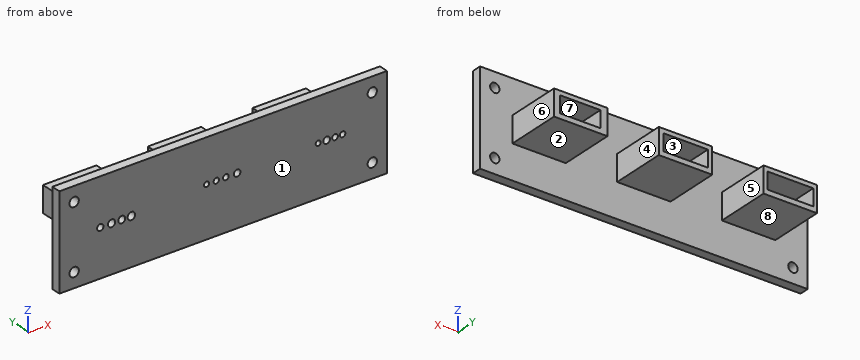
```python
from build123d import *

# Parameters (mm, degrees)
SKETCH1_W           = 88.9
SKETCH1_H           = 25.4
BOSS_EXTRUDE1_DEPTH = 2.54
SKETCH2_R           = 1.27
CUT_EXTRUDE1_DEPTH  = 2.54
SKETCH16_W          = 14.499999956
SKETCH16_H          = 6.99999997
BOSS_EXTRUDE3_DEPTH = 14.999999972
SKETCH17_W          = 12.390836481
SKETCH17_H          = 4.505758721
SKETCH17_W_2        = 12.015356588
SKETCH17_W_3        = 10.95149689
CUT_EXTRUDE4_DEPTH  = 12.459999972
SKETCH18_R          = 0.865438392
SKETCH18_R_2        = 0.972006337
SKETCH18_R_3        = 0.938699733
SKETCH18_R_4        = 1.023043952
SKETCH18_R_5        = 0.699865796
SKETCH18_R_6        = 0.72485584
SKETCH18_R_7        = 0.753208606
SKETCH18_R_8        = 0.89391984
SKETCH18_R_9        = 0.684371717
SKETCH18_R_10       = 0.906595882
SKETCH18_R_11       = 0.774291856
SKETCH18_R_12       = 0.739788643
CUT_EXTRUDE5_DEPTH  = 12.459999972


with BuildPart() as part:
    # Sketch1 → Boss-Extrude1 (new body)
    with BuildSketch(Plane(origin=(0, 0, 0), x_dir=(1, 0, 0), z_dir=(0, 1, 0))):
        Rectangle(SKETCH1_W, SKETCH1_H)
    extrude(amount=BOSS_EXTRUDE1_DEPTH)

    # Sketch2 → Cut-Extrude1 (cut)
    with BuildSketch(Plane(origin=(0, 2.54, 0), x_dir=(1, 0, 0), z_dir=(0, 1, 0))):
        with Locations((-40.45, 8.7)):
            Circle(SKETCH2_R)
        with Locations((-40.45, -8.7)):
            Circle(SKETCH2_R)
        with Locations((40.45, -8.7)):
            Circle(SKETCH2_R)
        with Locations((40.45, 8.7)):
            Circle(SKETCH2_R)
    extrude(amount=-CUT_EXTRUDE1_DEPTH, mode=Mode.SUBTRACT)

    # Sketch16 → Boss-Extrude3 (add)
    with BuildSketch(Plane(origin=(0, 2.54, 0), x_dir=(1, 0, 0), z_dir=(0, 1, 0))):
        Rectangle(SKETCH16_W, SKETCH16_H)
        with Locations((28.430000036, 1.27e-07)):
            Rectangle(SKETCH16_W, SKETCH16_H)
        with Locations((-28.430000036, 1.27e-07)):
            Rectangle(SKETCH16_W, SKETCH16_H)
    extrude(amount=BOSS_EXTRUDE3_DEPTH)

    # Sketch17 → Cut-Extrude4 (cut)
    with BuildSketch(Plane(origin=(0, 17.539999972, 0), x_dir=(1, 0, 0), z_dir=(0, 1, 0))):
        with Locations((-28.473891916, -0.093869973)):
            Rectangle(SKETCH17_W, SKETCH17_H)
        with Locations((-0.062579982, -0.093869973)):
            Rectangle(SKETCH17_W_2, SKETCH17_H)
        with Locations((28.567761889, -0.093869973)):
            Rectangle(SKETCH17_W_3, SKETCH17_H)
    extrude(amount=-CUT_EXTRUDE4_DEPTH, mode=Mode.SUBTRACT)

    # Sketch18 → Cut-Extrude5 (cut)
    with BuildSketch(Plane(origin=(0, 5.08, 0), x_dir=(1, 0, 0), z_dir=(0, 1, 0))):
        with Locations((-33.35513053, 0)):
            Circle(SKETCH18_R)
        with Locations((-30.2887114, 0)):
            Circle(SKETCH18_R_2)
        with Locations((-27.535192182, 0)):
            Circle(SKETCH18_R_3)
        with Locations((-24.906832928, 0)):
            Circle(SKETCH18_R_4)
        with Locations((-4.506191176, -1.023043952)):
            Circle(SKETCH18_R_5)
        with Locations((-1.873685579, -1.023043952)):
            Circle(SKETCH18_R_6)
        with Locations((0.727684736, -1.023043952)):
            Circle(SKETCH18_R_7)
        with Locations((3.790367697, -1.023043952)):
            Circle(SKETCH18_R_8)
        with Locations((25.783303286, -1.023043952)):
            Circle(SKETCH18_R_9)
        with Locations((28.074005802, -1.023043952)):
            Circle(SKETCH18_R_10)
        with Locations((30.354212641, -1.023043952)):
            Circle(SKETCH18_R_11)
        with Locations((32.413417846, -1.023043952)):
            Circle(SKETCH18_R_12)
    extrude(amount=-CUT_EXTRUDE5_DEPTH, mode=Mode.SUBTRACT)


solid = part.part
```
The model under review builds one solid part; all positions refer to its coordinate system, in mm. Face numbers are marked on the shaded views. A direction names the side the tool comes from. Coordinates: 2 decimals unless noted, no trailing zeros. Order: outer loops, then holes, each group sorted by start corner. A loop starts at its lowest first (then second) coordinate and runs counter-clockwise, first axis right, second up. Notation, with made-up numbers: (6.5, -33.75) -> (17.5, -33.75) arc R18 ccw to (17.5, -8.75) -> close; hole circle Ø11 at (-37, 55). An arc over 180 degrees is marked (long way). Answer in a Markdown table with one row per item. Add a question column.
Item 1: We need section D-D on x = 11. Write out the cut boundary in (y, z), plus the area to 3 significant figures.
Item 2: Machinability: for the marked faces 1, 2, 3 and 4, which of the approach directions +Z, -Z, +X, -X, +Y, -Y give a long, thin tool a straight path to every point of the face, cutting with its end or side? Answer none if there is none.
Item 3: We need section C-C on z = -8.7. Write out the cut boundary in (x, y), plus the area to 3 significant figures.
Item 4: Clearance check with flat-ended pins moving along their axes: pin 1 (6 mm diameter, centred on x = -28.5, y = 13, fed in from +Z); pin 2 (10 mm diameter, centred on x = -23, y = 11.5, fed in from -Z); pin 3 (5.5 mm diameter, centred on y = 7.5, z = -0.5, fed in from +X). State where each tip first meets the part, or that it passes through.
Item 5: To check wall thickness, follow probe 1 along X at (y, z) = (11.5, -1.75); probe 2 along X at (y, z) = (7.25, 2.75); probe 3 along X at (y, z) = (1.95, 8.7). State the ranges of each line that lie inside material, in increasing order.
Item 6: Mouldability with a two-part tool opening along X and no side actions: class the marked faces 5, 6, 7 and 8 as +X half, -X half, draft (parallel to the pull), parting line (faces both ways), or undercut.
Item 7: We need section A-A on y = 7. Write out the cut boundary in (x, z).
Item 8: We need section B-B on x = 40.45. Write out the cut boundary in (y, z), plus the area to 3 significant figures.
Final values:
| question | item | result |
|---|---|---|
| 1 | outline | (0, -12.7) -> (2.54, -12.7) -> (2.54, 12.7) -> (0, 12.7) -> close |
| 1 | area | 64.5 mm2 |
| 2 | face 1 | +Z, -Z, +X, -X, -Y |
| 2 | face 2 | -Z, +X, -X, +Y |
| 2 | face 3 | +Y |
| 2 | face 4 | +Z, -Z, +Y |
| 3 | outline | (-44.45, 0) -> (-41.72, 0) -> (-41.72, 2.54) -> (-44.45, 2.54) -> close; (-39.18, 0) -> (39.18, 0) -> (39.18, 2.54) -> (-39.18, 2.54) -> close; (41.72, 0) -> (44.45, 0) -> (44.45, 2.54) -> (41.72, 2.54) -> close |
| 3 | area | 213 mm2 |
| 4 | pin 1 | stops at z = 3.5 |
| 4 | pin 2 | stops at z = -3.5 |
| 4 | pin 3 | stops at x = 35.68 |
| 5 | probe 1 | x = -35.68 to -34.67, -22.28 to -21.18, -7.25 to -6.07, 5.95 to 7.25, 21.18 to 23.09, 34.04 to 35.68 |
| 5 | probe 2 | x = -35.68 to -21.18, -7.25 to 7.25, 21.18 to 35.68 |
| 5 | probe 3 | x = -44.45 to -41.72, -39.18 to 39.18, 41.72 to 44.45 |
| 6 | face 5 | undercut |
| 6 | face 6 | +X half |
| 6 | face 7 | undercut |
| 6 | face 8 | draft |
| 7 | outline | (-35.68, -3.5) -> (-21.18, -3.5) -> (-21.18, 3.5) -> (-35.68, 3.5) -> close; (-7.25, -3.5) -> (7.25, -3.5) -> (7.25, 3.5) -> (-7.25, 3.5) -> close; (21.18, -3.5) -> (35.68, -3.5) -> (35.68, 3.5) -> (21.18, 3.5) -> close; hole (-34.67, -2.16) -> (-22.28, -2.16) -> (-22.28, 2.35) -> (-34.67, 2.35) -> close; hole (-6.07, -2.16) -> (5.95, -2.16) -> (5.95, 2.35) -> (-6.07, 2.35) -> close; hole (23.09, -2.16) -> (34.04, -2.16) -> (34.04, 2.35) -> (23.09, 2.35) -> close |
| 8 | outline | (0, -12.7) -> (2.54, -12.7) -> (2.54, -9.97) -> (0, -9.97) -> close; (0, -7.43) -> (2.54, -7.43) -> (2.54, 7.43) -> (0, 7.43) -> close; (0, 9.97) -> (2.54, 9.97) -> (2.54, 12.7) -> (0, 12.7) -> close |
| 8 | area | 51.6 mm2 |
